The model under review builds one solid part; all positions refer to its coordinate system, in mm. A direction names the side the tool comes from. Round coordinates to 2 decimals unless told otherwise and drop trailing zeros. Write each loop counter-clockwise with the first axis right and the second up, starting at its lowest first coordinate (ties: lowest second). Pieces come first, ordered by that corner, then holes. Notation, with made-up numbers: (78, -4) - (125, -4) arc R16 cw to (125, 18) - close; hole circle Ø11 at (-19, 31). An arc over 180 degrees is marked (long way). Use one line per item in the form item = value.
from build123d import *

# Parameters (mm, degrees)
SKETCH1_W           = 40.386
SKETCH1_H           = 39.878
BOSS_EXTRUDE1_DEPTH = 20.32
SKETCH2_R           = 2.9464
BOSS_EXTRUDE2_DEPTH = 5.08
SKETCH3_W           = 3.175
SKETCH3_H           = 20.32
BOSS_EXTRUDE3_DEPTH = 7.62
SKETCH4_W           = 3.175
SKETCH4_H           = 20.32
BOSS_EXTRUDE4_DEPTH = 7.62
SKETCH5_R           = 2.2225
CUT_EXTRUDE1_DEPTH  = 60.854602831
SKETCH6_R           = 1.5875
CUT_EXTRUDE2_DEPTH  = 6.35
SKETCH7_R           = 2.2225
CUT_EXTRUDE3_DEPTH  = 60.854602831


with BuildPart() as part:
    # Sketch1 → Boss-Extrude1 (new body)
    with BuildSketch(Plane.XY):
        with Locations((20.193, 19.939)):
            Rectangle(SKETCH1_W, SKETCH1_H)
    extrude(amount=BOSS_EXTRUDE1_DEPTH)

    # Sketch2 → Boss-Extrude2 (add)
    with BuildSketch(Plane.ZY):
        with Locations(Location((10.16, 30.607, 0), (0, 0, 90))):
            Circle(SKETCH2_R)
    extrude(amount=BOSS_EXTRUDE2_DEPTH)

    # Sketch3 → Boss-Extrude3 (add)
    with BuildSketch(Plane(origin=(0, 39.878, 0), x_dir=(1, 0, 0), z_dir=(0, 1, 0))):
        with Locations((11.7475, -10.16)):
            Rectangle(SKETCH3_W, SKETCH3_H)
    extrude(amount=BOSS_EXTRUDE3_DEPTH)

    # Sketch4 → Boss-Extrude4 (add)
    with BuildSketch(Plane.XZ):
        with Locations((11.7475, 10.16)):
            Rectangle(SKETCH4_W, SKETCH4_H)
    extrude(amount=BOSS_EXTRUDE4_DEPTH)

    # Sketch5 → Cut-Extrude1 (cut, through all)
    with BuildSketch(Plane.ZY.offset(-10.16)):
        with Locations((5.207, 44.6405)):
            Circle(SKETCH5_R)
        with Locations((15.113, 44.6405)):
            Circle(SKETCH5_R)
    extrude(amount=-CUT_EXTRUDE1_DEPTH, mode=Mode.SUBTRACT)

    # Sketch6 → Cut-Extrude2 (cut)
    with BuildSketch(Plane.ZY.offset(5.08)):
        with Locations((10.16, 30.607)):
            Circle(SKETCH6_R)
    extrude(amount=-CUT_EXTRUDE2_DEPTH, mode=Mode.SUBTRACT)

    # Sketch7 → Cut-Extrude3 (cut, through all)
    with BuildSketch(Plane.ZY.offset(-10.16)):
        with Locations((15.113, -4.7625)):
            Circle(SKETCH7_R)
        with Locations((5.207, -4.7625)):
            Circle(SKETCH7_R)
    extrude(amount=-CUT_EXTRUDE3_DEPTH, mode=Mode.SUBTRACT)


solid = part.part
(1) Add section D-D on x = 36. Write out the cut boundary in (y, z).
Geometry results:
outline = (0, 0) - (39.88, 0) - (39.88, 20.32) - (0, 20.32) - close
(2) To check wall thickness, follow L1, parallel to Y at x = -3.5, z = 10.16; L2, parallel to X at y = 31, z = 13.5; L3, parallel to X at y = 31.5, z = 9.75. State the ranges of each line that lie inside material, in increasing order.
Geometry results:
L1 = 27.66 to 29.02, 32.19 to 33.55
L2 = 0 to 40.39
L3 = 1.27 to 40.39
(3) Add section A-A on z = 10.16. Write out the cut boundary in (x, y) (1 decimal), then the cut area to 3 significant figures.
Geometry results:
outline = (-5.1, 27.7) - (0, 27.7) - (0, 0) - (10.2, 0) - (10.2, -7.6) - (13.3, -7.6) - (13.3, 0) - (40.4, 0) - (40.4, 39.9) - (13.3, 39.9) - (13.3, 47.5) - (10.2, 47.5) - (10.2, 39.9) - (0, 39.9) - (0, 33.6) - (-5.1, 33.6) - (-5.1, 32.2) - (1.3, 32.2) - (1.3, 29) - (-5.1, 29) - close
area = 1,670 mm2
(4) The part is to be moulded in two halves that separate along Z. For faces 5 (the cylindrical face through (11.73, 42.67, 16.14)), 6 (the flat face through (13.335, 44, 10)), 7 (the cylindrical face through (11.725, -6.734, 6.233)), 8 (the flat face through (20, 20, 0)), say which applies: +Z half, -Z half, draft (parallel to the pull), parting line (faces both ways), or undercut.
Geometry results:
face_5 = undercut
face_6 = draft
face_7 = undercut
face_8 = -Z half
(5) Machinability: for faces 1 (the flat face through (10.16, -4, 10)), 2 (the flat face through (10.16, 44, 10)), 3 (the flat face through (1.27, 31, 10)), 4 (the flat face through (27, 0, 10)), which of the approach directions +Z, -Z, +X, -X, +Y, -Y give a long, thin tool a straight path to every point of the face, cutting with its end or side? Answer none if there is none.
Geometry results:
face_1 = +Z, -Z, -X, -Y
face_2 = +Z, -Z, -X, +Y
face_3 = -X
face_4 = +Z, -Z, +X, -Y
(6) Insertion check: P1, Ø6, axis at y = 37.5, z = 6.5, coming from the -X side; P2, Ø1, axis at y = 31, z = 10.5, coming from the -X side; P3, Ø2, axis at x = 10, z = 17, coming from the -Y side; P4, Ø6, axis at y = 44.64, z = 5.21, coming from the +X side (3 decimals). Each pin has a flat end and moves straight along its axis. Give the tip position at first contact, or say it passes through.
Geometry results:
P1 = 0
P2 = 1.27
P3 = -7.62
P4 = 13.335
(7) Add section B-B on z = 14.5. Write out the cut boundary in (x, y) (3 decimals).
Geometry results:
outline = (0, 0) - (10.16, 0) - (10.16, -2.626) - (13.335, -2.626) - (13.335, 0) - (40.386, 0) - (40.386, 39.878) - (13.335, 39.878) - (13.335, 42.504) - (10.16, 42.504) - (10.16, 39.878) - (0, 39.878) - close; (10.16, -7.62) - (13.335, -7.62) - (13.335, -6.899) - (10.16, -6.899) - close; (10.16, 46.777) - (13.335, 46.777) - (13.335, 47.498) - (10.16, 47.498) - close
(8) Add section C-C on y = 15. Write out the cut boundary in (x, z).
Geometry results:
outline = (0, 0) - (40.39, 0) - (40.39, 20.32) - (0, 20.32) - close
